Design review of the part built by this model. Coordinates are the model's own, in mm. A direction names the side the tool comes from. Round coordinates to 2 decimals unless told otherwise and drop trailing zeros. Write each loop counter-clockwise with the first axis right and the second up, starting at its lowest first coordinate (ties: lowest second). Pieces come first, ordered by that corner, then holes.
from build123d import *

# Parameters (mm, degrees)
BOSS_EXTRUDE1_DEPTH = 25.4
CUT_EXTRUDE1_REACH  = 129.762
SKETCH3_R           = 3.175


with BuildPart() as part:
    # Sketch2 → Boss-Extrude1 (new body)
    with BuildSketch(Plane.XY):
        Polygon((0, 0), (12.7, 0), (12.7, -40.64), (66.04, -44.773379719), (114.3, -40.64), (114.3, -32.073379719), (111.76, -32.073379719), (111.76, -35.56), (66.04, -39.475833418), (19.05, -35.56), (19.05, 0), (19.05, 6.35), (0, 6.35), align=None)
        Polygon((-12.7, 0), (0, 0), (0, 6.35), (-19.05, 6.35), (-19.05, 0), (-19.05, -35.56), (-66.04, -39.475833418), (-111.76, -35.56), (-111.76, -32.073379719), (-114.3, -32.073379719), (-114.3, -40.64), (-66.04, -44.773379719), (-12.7, -40.64), align=None)
    extrude(amount=BOSS_EXTRUDE1_DEPTH)

    # Sketch3 → Cut-Extrude1 (cut, up to next)
    with BuildSketch(Plane(origin=(0, 6.35, 0), x_dir=(1, 0, 0), z_dir=(0, 1, 0)), mode=Mode.PRIVATE) as cut_extrude1_sk1:
        with Locations(Location((0, -12.7, 0), (0, 0, 180))):
            Circle(SKETCH3_R)
    cut_extrude1_tool1 = extrude(cut_extrude1_sk1.sketch, amount=-CUT_EXTRUDE1_REACH, mode=Mode.PRIVATE) & part.part
    add(cut_extrude1_tool1.solids().sort_by_distance((0, 6.35, 12.7))[0], mode=Mode.SUBTRACT)


solid = part.part
1) The part is to be moulded in two halves that separate along Z. For faces 1 (the face through (3, 0, 15)), 2 (the face through (-1.5, 3.2, 9.9)), 3 (the face through (-17, -27, 0)), say which applies: pulls with the +Z half, pulls with the -Z half, needs draft (parallel to the pull), parting line crosses it, or undercut.
2) For line 1 along X through (y, z) = (-32, 23.25); line 2 along Z through (x, y) = (0, 3) (3 decimals); line 3 along X through (y, z) = (-40.5, 22.5), list the stretches that pass through material, from the lowest coordinate up.
3) For faces 4 (the face through (-4, 6.35, 13)), 5 (the face through (42.874, -37.545, 12.522)), 6 (the face through (-39.743, -42.736, 12.522)), list the 3-axis set-ups (+Z, -Z, +X, -X, +Y, -Y) from which the entire face can be reached by the end or side of a thin tool; tool diameter is ignored.
4) For P1, Ø1.5, axis at y = -3, z = 16.5, coming from the +X side; P2, Ø5, axis at x = -35, z = 4.5, coming from the +Y side; P3, Ø5, axis at x = -60, z = 14, coming from the +Y side; P4, Ø12, axis at x = -64, y = -30.5, coming from the +Z side, all flat-tipped, find the tip position at first contact; note any pin that passes through.
5) Add section C-C on x = 0. State the section outline as (y, z) points (3 decimals), and give its area (3 significant figures).
6) Add section D-D on x = -61. State the section outline as (y, z) points.
7) Add section A-A on y = -24.5. State the section outline as (x, z) points.
8) Add section B-B on z = 12.7. State the section outline as (x, y) points (3 decimals).
Computed:
1. face 1: needs draft
1. face 2: undercut
1. face 3: pulls with the -Z half
2. line 1: x = -19.05 to -12.7, 12.7 to 19.05
2. line 2: z = 0 to 9.525, 15.875 to 25.4
2. line 3: x = -114.3 to -12.7, 12.7 to 114.3
3. face 4: +Z, -Z, +X, -X, +Y
3. face 5: +Z, -Z, +Y
3. face 6: +Z, -Z, -Y
4. P1: stops at x = 19.05
4. P2: stops at y = -36.68
4. P3: stops at y = -38.76
4. P4: passes through
5. outline: (0, 0) - (6.35, 0) - (6.35, 9.525) - (0, 9.525) - close; (0, 15.875) - (6.35, 15.875) - (6.35, 25.4) - (0, 25.4) - close
5. area: 121 mm2
6. outline: (-44.38, 0) - (-39.06, 0) - (-39.06, 25.4) - (-44.38, 25.4) - close
7. outline: (-19.05, 0) - (-12.7, 0) - (-12.7, 25.4) - (-19.05, 25.4) - close; (12.7, 0) - (19.05, 0) - (19.05, 25.4) - (12.7, 25.4) - close
8. outline: (-114.3, -40.64) - (-66.04, -44.773) - (-12.7, -40.64) - (-12.7, 0) - (-3.175, 0) - (-3.175, 6.35) - (-19.05, 6.35) - (-19.05, -35.56) - (-66.04, -39.476) - (-111.76, -35.56) - (-111.76, -32.073) - (-114.3, -32.073) - close; (3.175, 0) - (12.7, 0) - (12.7, -40.64) - (66.04, -44.773) - (114.3, -40.64) - (114.3, -32.073) - (111.76, -32.073) - (111.76, -35.56) - (66.04, -39.476) - (19.05, -35.56) - (19.05, 6.35) - (3.175, 6.35) - close
